```python
from build123d import *

# Parameters (mm, degrees)
BOSS_EXTRUDE1_DEPTH = 3
SKETCH3_R           = 1
CUT_EXTRUDE1_DEPTH  = 4


with BuildPart() as part:
    # Sketch1 → Boss-Extrude1 (new body)
    with BuildSketch(Plane(origin=(0, 0, 0), x_dir=(1, 0, 0), z_dir=(0, 1, 0))):
        with BuildLine():
            Line((27.034499206, -59.38314523), (27.034499206, -77.961788992))
            ThreePointArc((27.034499206, -77.961788992), (30.840522581, -97.095960611), (41.679160147, -113.317128052))
            Line((41.679160147, -113.317128052), (42.389838265, -114.02780617))
            ThreePointArc((42.389838265, -114.02780617), (58.611005706, -124.866443737), (77.745177325, -128.672467111))
            Line((77.745177325, -128.672467111), (156.323821087, -128.672467111))
            ThreePointArc((156.323821087, -128.672467111), (175.457992706, -124.866443737), (191.679160147, -114.02780617))
            Line((191.679160147, -114.02780617), (192.389838265, -113.317128052))
            ThreePointArc((192.389838265, -113.317128052), (203.228475832, -97.095960611), (207.034499206, -77.961788992))
            Line((207.034499206, -77.961788992), (207.034499206, -61.064291371))
            ThreePointArc((207.034499206, -61.064291371), (202.66744641, -40.628192686), (190.329134028, -23.761914877))
            Line((190.329134028, -23.761914877), (187.649401106, -21.370090617))
            ThreePointArc((187.649401106, -21.370090617), (172.171628737, -11.954596736), (154.354766284, -8.672467111))
            Line((154.354766284, -8.672467111), (77.745177325, -8.672467111))
            ThreePointArc((77.745177325, -8.672467111), (58.611005706, -12.478490485), (42.389838265, -23.317128052))
            Line((42.389838265, -23.317128052), (41.679160147, -24.02780617))
            ThreePointArc((41.679160147, -24.02780617), (30.840522581, -40.248973611), (27.034499206, -59.38314523))
        make_face()
    extrude(amount=BOSS_EXTRUDE1_DEPTH)

    # Sketch3 → Cut-Extrude1 (cut, through all)
    with BuildSketch(Plane(origin=(0, 3, 0), x_dir=(1, 0, 0), z_dir=(0, 1, 0))):
        with Locations((70.463718508, -40.729998692)):
            Circle(SKETCH3_R)
        with Locations((46.453916589, -26.324117541)):
            Circle(SKETCH3_R)
        with Locations((117.034499206, -41.672467111)):
            Circle(SKETCH3_R)
        with Locations((184.546793577, -25.302810972)):
            Circle(SKETCH3_R)
        with Locations((117.034499206, -13.672467111)):
            Circle(SKETCH3_R)
        with Locations((160.707496688, -39.989128545)):
            Circle(SKETCH3_R)
        with Locations((163.605279904, -96.61493553)):
            Circle(SKETCH3_R)
        with Locations((187.615081824, -111.020816682)):
            Circle(SKETCH3_R)
        with Locations((117.034499206, -95.672467111)):
            Circle(SKETCH3_R)
        with Locations((117.034499206, -123.672467111)):
            Circle(SKETCH3_R)
        with Locations((46.054672056, -110.621572149)):
            Circle(SKETCH3_R)
        with Locations((69.893968945, -95.935254577)):
            Circle(SKETCH3_R)
    extrude(amount=-CUT_EXTRUDE1_DEPTH, mode=Mode.SUBTRACT)


solid = part.part
```
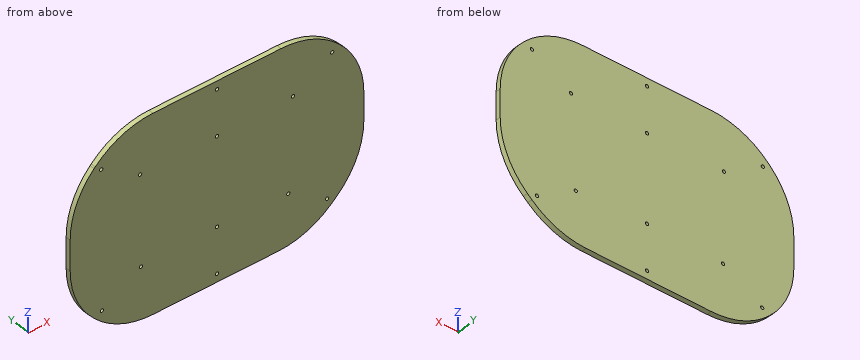
The model under review builds one solid part; all positions refer to its coordinate system, in mm. Round coordinates to 2 decimals unless told otherwise and drop trailing zeros. Order: outer loops, then holes, each group sorted by start corner. A loop starts at its lowest first (then second) coordinate and runs counter-clockwise, first axis right, second up. Notation, with made-up numbers: (2.25, -25) -> (30.25, -25) arc R12 cw to (30.25, -5) -> close; hole circle Ø5 at (66, 6). An arc over 180 degrees is marked (long way). One line per item, written item: value. Start each with the question number.
Q1. Take a section at C-C (x = 167). Write out the cut boundary in (y, z), and give its area (3 significant figures).
Q2. Take a section at A-A (y = 0.45). Count the separate pieces of the cut face and the enclosed holes in it, and give its area (3 significant figures).
Q3. Take a section at B-B (x = 50.5). Write out the cut boundary in (y, z).
Q4. Clearance check with a flat-ended pin moving along its axis: pin 1 Ø1.6 at (x, z) = (163.61, 96.61) entering from -Y. State where the tip first meets the part, or that it passes through.
Q5. Wall thickness on line 1 (X direction, y = 0.8, z = 111); line 2 (Z direction, x = 71, y = 0.95); line 3 (X direction, y = 2.4, z = 19.5): over which ranges is each line inside the solid? List them lowest first.
Reported:
1. outline: (0, 10.3) -> (3, 10.3) -> (3, 127.52) -> (0, 127.52) -> close
1. area: 352 mm2
2. separate pieces: 1
2. enclosed holes: 12
2. area: 19,300 mm2
3. outline: (0, 16.75) -> (3, 16.75) -> (3, 120.6) -> (0, 120.6) -> close
4. pin 1: passes through
5. line 1: x = 39.5 to 45.13, 46.98 to 186.62, 188.61 to 194.56
5. line 2: z = 9.13 to 39.89, 41.57 to 128.22
5. line 3: x = 46.67 to 185.43
